```python
from build123d import *

# Parameters (mm, degrees)
EXTRUDE_1_DEPTH        = 10
HOLE_WIZARD_M6_1_D     = 5
HOLE_WIZARD_M6_1_DEPTH = 15
HOLE_WIZARD_M6_1_TIP   = 1.502151548


with BuildPart() as part:
    # 草图1 → 凸台-拉伸1 (new, symmetric)
    with BuildSketch(Plane.XY):
        with BuildLine():
            Line((-0.162211674, 0.146446609), (-2.819318456, 2.803553391))
            ThreePointArc((-2.819318456, 2.803553391), (-2.927704831, 2.965765065), (-2.965765065, 3.157106781))
            Line((-2.965765065, 3.157106781), (-2.965765065, 5.8))
            ThreePointArc((-2.965765065, 5.8), (-2.819318456, 6.153553391), (-2.465765065, 6.3))
            Line((-2.465765065, 6.3), (-0.015765065, 6.3))
            Line((-0.015765065, 6.3), (-0.015765065, 9.2))
            ThreePointArc((-0.015765065, 9.2), (0.130681544, 9.553553391), (0.484234935, 9.7))
            Line((0.484234935, 9.7), (3.384234935, 9.7))
            Line((3.384234935, 9.7), (3.884234935, 8.9))
            Line((3.884234935, 8.9), (4.384234935, 9.7))
            Line((4.384234935, 9.7), (7.284234935, 9.7))
            ThreePointArc((7.284234935, 9.7), (7.637788326, 9.553553391), (7.784234935, 9.2))
            Line((7.784234935, 9.2), (7.784234935, 6.3))
            Line((7.784234935, 6.3), (10.234234935, 6.3))
            ThreePointArc((10.234234935, 6.3), (10.587788326, 6.153553391), (10.734234935, 5.8))
            Line((10.734234935, 5.8), (10.734234935, 3.157106781))
            ThreePointArc((10.734234935, 3.157106781), (10.696174701, 2.965765065), (10.587788326, 2.803553391))
            Line((10.587788326, 2.803553391), (7.930681544, 0.146446609))
            ThreePointArc((7.930681544, 0.146446609), (7.76846987, 0.038060234), (7.577128154, 0))
            Line((7.577128154, 0), (0.191341716, 0))
            ThreePointArc((0.191341716, 0), (0, 0.038060234), (-0.162211674, 0.146446609))
        make_face()
    extrude(amount=EXTRUDE_1_DEPTH, both=True)

    # M6 螺纹孔1
    with Locations(Plane(origin=(3.884234935, 0, 0), x_dir=(-1, 0, 0), z_dir=(0, -1, 0))):
        with Locations((0, 0)):
            Hole(HOLE_WIZARD_M6_1_D / 2, depth=HOLE_WIZARD_M6_1_DEPTH)
            with Locations((0, 0, -(HOLE_WIZARD_M6_1_DEPTH + HOLE_WIZARD_M6_1_TIP / 2))):  # 118° drill point
                Cone(0, HOLE_WIZARD_M6_1_D / 2, HOLE_WIZARD_M6_1_TIP, mode=Mode.SUBTRACT)


solid = part.part
```
Here's how the part is built. I have some questions about the finished solid (model axes, mm). A direction names the side the tool comes from. Give positions to 0.01 mm unless a question says otherwise; leave off trailing zeros. Order: outer loops, then holes, each group sorted by start corner. A loop starts at its lowest first (then second) coordinate and runs counter-clockwise, first axis right, second up. Notation, with made-up numbers: (68, 67) - (72, 67) arc R11 cw to (72, 86) - close; hole circle Ø1 at (64, -25.75). An arc over 180 degrees is marked (long way). Answer as a JSON object with one key per item and string values. Group by question number.
Item 1: If we section it at D-D on x = 2: Please give me the cut outline in (y, z), and give its area (3 significant figures).
Item 2: Please list where these lines run through material, in increasing order: probe 1 along Z at (x, y) = (4, 6); probe 2 along X at (y, z) = (8.75, 0.75); probe 3 along Z at (x, y) = (5.5, 4.5).
Item 3: If we section it at B-B on x = 5.75: Please give me the cut outline in (y, z).
Item 4: If we mould it in two halves opening along X, with no side actions, what happens to faces 4 (the flat face through (3.63, 9.31, 6.28)), 5 (the flat face through (1, 9.7, 0)), 6 (the flat face through (-2.966, 4, 0))? For each: pulls with the +X half, pulls with the -X half, needs draft (parallel to the pull), parting line crosses it, or undercut.
Item 5: If we section it at A-A on z = 0: Please give me the cut outline in (x, y), and give its area (3 significant figures).
Item 6: Which directions (+Z, -Z, +X, -X, +Y, -Y) give clear straight access to the entire face, cutting with the end or side of a thin tool? Please do faces 1 (the flat face through (7.784, 8, 0)), 2 (the flat face through (-1.472, 1.456, 0.14)), 3 (the flat face through (-1, 6.3, 0)).
Item 7: For P1, Ø2.5, axis at y = 8.5, z = -4, coming from the +X side; P2, Ø1.2, axis at x = 8.5, z = -2.5, coming from the +Y side; P3, Ø0.9, axis at y = 7, z = -2.5, coming from the -X side, each with a flat end and sliding along its axis, tell me the tip position at first contact or that it passes through.
Item 8: If we section it at C-C on z = -6.25: Please give me the cut outline in (x, y), and give its area (3 significant figures).
Result set:
{
 "1": {"outline": "(0, -10) - (9.7, -10) - (9.7, -1.64) - (0, -1.64) - close; (0, 1.64) - (9.7, 1.64) - (9.7, 10) - (0, 10) - close", "area": "162 mm²"},
 "2": {"probe 1": "-10 to -2.5, 2.5 to 10", "probe 2": "-0.02 to 1.5, 6.27 to 7.78", "probe 3": "-10 to -1.91, 1.91 to 10"},
 "3": {"outline": "(0, -10) - (9.7, -10) - (9.7, -1.66) - (0, -1.66) - close; (0, 1.66) - (9.7, 1.66) - (9.7, 10) - (0, 10) - close"},
 "4": {"face 4": "undercut", "face 5": "needs draft", "face 6": "pulls with the -X half"},
 "5": {"outline": "(-2.97, 3.16) arc R0.5 ccw to (-2.82, 2.8) - (-0.16, 0.15) arc R0.5 ccw to (0.19, 0) - (1.38, 0) - (1.38, 9.7) - (0.48, 9.7) arc R0.5 ccw to (-0.02, 9.2) - (-0.02, 6.3) - (-2.47, 6.3) arc R0.5 ccw to (-2.97, 5.8) - close; (6.38, 0) - (7.58, 0) arc R0.5 ccw to (7.93, 0.15) - (10.59, 2.8) arc R0.5 ccw to (10.73, 3.16) - (10.73, 5.8) arc R0.5 ccw to (10.23, 6.3) - (7.78, 6.3) - (7.78, 9.2) arc R0.5 ccw to (7.28, 9.7) - (6.38, 9.7) - close", "area": "55.4 mm²"},
 "6": {"face 1": "+Z, -Z, +X, +Y", "face 2": "+Z, -Z, -X, -Y", "face 3": "+Z, -Z, -X, +Y"},
 "7": {"P1": "x = 7.78", "P2": "y = 6.3", "P3": "x = -0.02"},
 "8": {"outline": "(-2.97, 3.16) arc R0.5 ccw to (-2.82, 2.8) - (-0.16, 0.15) arc R0.5 ccw to (0.19, 0) - (7.58, 0) arc R0.5 ccw to (7.93, 0.15) - (10.59, 2.8) arc R0.5 ccw to (10.73, 3.16) - (10.73, 5.8) arc R0.5 ccw to (10.23, 6.3) - (7.78, 6.3) - (7.78, 9.2) arc R0.5 ccw to (7.28, 9.7) - (4.38, 9.7) - (3.88, 8.9) - (3.38, 9.7) - (0.48, 9.7) arc R0.5 ccw to (-0.02, 9.2) - (-0.02, 6.3) - (-2.47, 6.3) arc R0.5 ccw to (-2.97, 5.8) - close", "area": "103 mm²"}
}
